For this review, take the finished solid that the model builds, in its own axes (mm). Give positions to 0.01 mm unless a question says otherwise; leave off trailing zeros. Loops run counter-clockwise (first coordinate to the right, second up) from the corner with the lowest first, then second, coordinate; pieces in that order, holes last. Notation, with made-up numbers: (45.5, 85) - (101.5, 85) arc R20 cw to (101.5, 110) - close; hole circle Ø9 at (-34.75, 36.5). An arc over 180 degrees is marked (long way). Put each result on its own line as item: value.
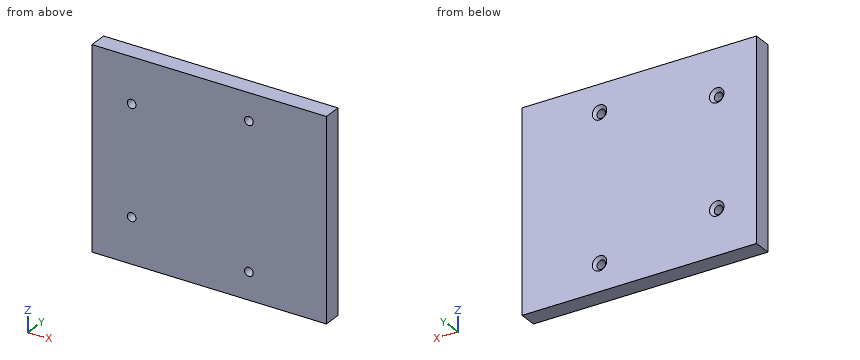
from build123d import *

# Parameters (mm, degrees)
SKETCH_2_W      = 130
SKETCH_2_H      = 110
SKETCH_2_R      = 2.4
EXTRUDE_1_DEPTH = 5
CHAMFER_1_SIZE  = 1.6


with BuildPart() as part:
    # Эскиз2 → Бобышка-Вытянуть1 (new, symmetric)
    with BuildSketch(Plane(origin=(0, 0, 0), x_dir=(1, 0, 0), z_dir=(0, 1, 0))):
        Rectangle(SKETCH_2_W, SKETCH_2_H)
        with Locations(Location((-43, 30, 0), (0, 0, 270))):
            Circle(SKETCH_2_R, mode=Mode.SUBTRACT)
        with Locations(Location((-43, -30, 0), (0, 0, 270))):
            Circle(SKETCH_2_R, mode=Mode.SUBTRACT)
        with Locations(Location((22, 40, 0), (0, 0, 270))):
            Circle(SKETCH_2_R, mode=Mode.SUBTRACT)
        with Locations(Location((22, -40, 0), (0, 0, 270))):
            Circle(SKETCH_2_R, mode=Mode.SUBTRACT)
    extrude(amount=EXTRUDE_1_DEPTH, both=True)

    # Фаска1
    chamfer_1_edges = [part.edges().sort_by_distance(p)[0] for p in [
        (-43, 5, -32.4),
        (-43, 5, 27.6),
        (22, 5, -42.4),
        (22, 5, 37.6),
    ]]
    chamfer(chamfer_1_edges, length=CHAMFER_1_SIZE)


solid = part.part
1) Insertion check: pin 1 Ø6 at (x, z) = (22, -40) entering from +Y; pin 2 Ø4 at (x, z) = (-43, 30) entering from +Y. Each pin has a flat end and moves straight along its axis. Give the tip position at first contact, or say it passes through.
Geometry check:
pin 1: stops at y = 4
pin 2: passes through
2) Wall thickness on line 1 (X direction, y = 0, z = 30); line 2 (X direction, y = 0.25, z = 40); line 3 (Z direction, x = -44, y = -2): over which ranges is each line inside the solid? List them lowest first.
Geometry check:
line 1: x = -65 to -45.4, -40.6 to 65
line 2: x = -65 to 19.6, 24.4 to 65
line 3: z = -55 to -32.18, -27.82 to 27.82, 32.18 to 55
3) Take a section at A-A on x = 22. State the section outline as (y, z) points.
Geometry check:
outline: (-5, -55) - (5, -55) - (5, -44) - (3.4, -42.4) - (-5, -42.4) - close; (-5, -37.6) - (3.4, -37.6) - (5, -36) - (5, 36) - (3.4, 37.6) - (-5, 37.6) - close; (-5, 42.4) - (3.4, 42.4) - (5, 44) - (5, 55) - (-5, 55) - close
4) Take a section at B-B on z = 40. State the section outline as (x, y) points.
Geometry check:
outline: (-65, -5) - (19.6, -5) - (19.6, 3.4) - (18, 5) - (-65, 5) - close; (24.4, -5) - (65, -5) - (65, 5) - (26, 5) - (24.4, 3.4) - close
